```python
from build123d import *

# Parameters (mm, degrees)
SKETCH1_W           = 40.954999878
SKETCH1_H           = 27.518000082
BOSS_EXTRUDE1_DEPTH = 2.999994
SKETCH3_W           = 20.955
SKETCH3_H           = 7.5184
BOSS_EXTRUDE2_DEPTH = 21.874999989
SKETCH4_R           = 1.999996
CUT_EXTRUDE1_DEPTH  = 3.999994
SKETCH5_R           = 6.6675
CUT_EXTRUDE2_DEPTH  = 2.54
SKETCH6_R           = 8.0645
CUT_EXTRUDE3_DEPTH  = 4.9784


with BuildPart() as part:
    # Sketch1 → Boss-Extrude1 (new body)
    with BuildSketch(Plane(origin=(0, 0, 0), x_dir=(1, 0, 0), z_dir=(0, 1, 0))):
        with Locations((20.477499939, 13.759000041)):
            Rectangle(SKETCH1_W, SKETCH1_H)
    extrude(amount=-BOSS_EXTRUDE1_DEPTH)

    # Sketch3 → Boss-Extrude2 (add)
    with BuildSketch(Plane(origin=(0, 0, 0), x_dir=(1, 0, 0), z_dir=(0, 1, 0))):
        with Locations((21.4775034, 14.7592034)):
            Rectangle(SKETCH3_W, SKETCH3_H)
    extrude(amount=BOSS_EXTRUDE2_DEPTH)

    # Sketch4 → Cut-Extrude1 (cut, through all)
    with BuildSketch(Plane(origin=(0, 0, 0), x_dir=(1, 0, 0), z_dir=(0, 1, 0))):
        with Locations((2.999994, 24.518006082)):
            Circle(SKETCH4_R)
        with Locations((2.999994, 2.999994)):
            Circle(SKETCH4_R)
        with Locations((37.955005756, 2.999994)):
            Circle(SKETCH4_R)
        with Locations((37.955005756, 24.518006082)):
            Circle(SKETCH4_R)
    extrude(amount=-CUT_EXTRUDE1_DEPTH, mode=Mode.SUBTRACT)

    # Sketch5 → Cut-Extrude2 (cut)
    with BuildSketch(Plane.XY.offset(-11.0000034)):
        with Locations((21.4775034, 10.843006)):
            Circle(SKETCH5_R)
    extrude(amount=-CUT_EXTRUDE2_DEPTH, mode=Mode.SUBTRACT)

    # Sketch6 → Cut-Extrude3 (cut)
    with BuildSketch(Plane(origin=(0, 0, -18.5184034), x_dir=(-1, 0, 0), z_dir=(0, 0, -1))):
        with Locations((-21.4775034, 10.843006)):
            Circle(SKETCH6_R)
    extrude(amount=-CUT_EXTRUDE3_DEPTH, mode=Mode.SUBTRACT)


solid = part.part
```
For this review, take the finished solid that the model builds, in its own axes (mm). A direction names the side the tool comes from. Round coordinates to 2 decimals unless told otherwise and drop trailing zeros. Order: outer loops, then holes, each group sorted by start corner. A loop starts at its lowest first (then second) coordinate and runs counter-clockwise, first axis right, second up.
Q1. We need section D-D, the plane z = -15.25. Give the boundary of the cut face in (x, y) (1 decimal).
Findings below:
outline: (0, -3) - (41, -3) - (41, 0) - (32, 0) - (32, 21.9) - (11, 21.9) - (11, 0) - (0, 0) - close; hole circle Ø16.1 at (21.5, 10.8)
Q2. We need section A-A, the plane z = -23.25. Give the boundary of the cut face in (x, y) (3 decimals), plus the area to 3 significant figures.
Findings below:
outline: (0, -3) - (1.453, -3) - (1.453, 0) - (0, 0) - close; (4.547, -3) - (36.408, -3) - (36.408, 0) - (4.547, 0) - close; (39.502, -3) - (40.955, -3) - (40.955, 0) - (39.502, 0) - close
area: 104 mm2
Q3. We need section C-C, the plane y = 7. Give the boundary of the cut face in (x, z) (3 decimals), plus the area to 3 significant figures.
Findings below:
outline: (11, -18.518) - (14.388, -18.518) - (14.388, -13.54) - (16.029, -13.54) - (16.029, -11) - (11, -11) - close; (26.926, -13.54) - (28.567, -13.54) - (28.567, -18.518) - (31.955, -18.518) - (31.955, -11) - (26.926, -11) - close
area: 59.3 mm2
Q4. Mouldability with a two-part tool opening along X and no side actions: class faces 1 (the cylindrical face through (39.8, -1.48, -2.23)), 2 (the flat face through (20, -1, -27.518)), 3 (the flat face through (40.955, -1, -14)), 4 (the cylindrical face through (2.74, -1.48, -26.5)) as pulls with the +X half, pulls with the -X half, needs draft (parallel to the pull), parting line crosses it, or undercut.
Findings below:
face 1: undercut
face 2: needs draft
face 3: pulls with the +X half
face 4: undercut
Q5. Wall thickness on line 1 (Y direction, x = 9, z = -3.5); line 2 (X direction, y = 12, z = -13.25) (3 decimals); line 3 (Y direction, x = 17, z = -15) (3 decimals): over which ranges is each line inside the solid? List them lowest first.
Findings below:
line 1: y = -3 to 0
line 2: x = 11 to 14.911, 28.044 to 31.955
line 3: y = -3 to 4.136, 17.55 to 21.875
Q6. We need section B-B, the plane x = 23. Give the boundary of the cut face in (y, z) (3 decimals), plus the area to 3 significant figures.
Findings below:
outline: (-3, -27.518) - (0, -27.518) - (0, -18.518) - (2.924, -18.518) - (2.924, -13.54) - (4.352, -13.54) - (4.352, -11) - (0, -11) - (0, 0) - (-3, 0) - close; (17.334, -13.54) - (18.762, -13.54) - (18.762, -18.518) - (21.875, -18.518) - (21.875, -11) - (17.334, -11) - close
area: 135 mm2
Q7. Machinability: for faces 5 (the flat face through (14, 6, -18.518)), 6 (the flat face through (11, 11, -15)), 7 (the flat face through (31.955, 11, -15)), 8 (the flat face through (16.7, 5.9, -11)), which of the approach directions +Z, -Z, +X, -X, +Y, -Y give a long, thin tool a straight path to every point of the face, cutting with its end or side? Answer none if there is none.
Findings below:
face 5: -Z, +X, -X, +Y
face 6: +Z, -Z, -X, +Y
face 7: +Z, -Z, +X, +Y
face 8: +Z, +X, -X, +Y
Q8. Insertion check: P1, Ø10, axis at x = 16.5, y = 7.5, coming from the -Z side; P2, Ø8.5, axis at y = 11.5, z = -15.5, coming from the +X side (3 decimals); P3, Ø3, axis at x = 23, z = -24.5, coming from the +Y side. Each pin has a flat end and moves straight along its axis. Give the tip position at first contact, or say it passes through.
Findings below:
P1: stops at z = -18.52
P2: stops at x = 31.955
P3: stops at y = 0
